Geometry: final body of the model. Coordinates: model frame, mm. A direction names the side the tool comes from. Coordinates: 2 decimals unless noted, no trailing zeros. Loops run counter-clockwise (first coordinate to the right, second up) from the corner with the lowest first, then second, coordinate; pieces in that order, holes last. Notation, with made-up numbers: (-24.5, 50) - (29.5, 50) arc R25 ccw to (29.5, 73) - close; hole circle Ø3 at (82, 30). An arc over 180 degrees is marked (long way). Put each result on its own line as item: value. Start each with the question number.
1) Reachability of faces 1 (the flat face through (-4, 4, -4)), 2 (the flat face through (0, 4, 17.5)) from +Z, -Z, +X, -X, +Y, -Y: full face, straight path, thin tool, end or side. Return the list, or none.
2) Material intervals for line 1 along Z through (x, y) = (13.5, 7); line 2 along Z through (x, y) = (-16, 5.75); line 3 along X through (y, z) = (3, -27), sorted ascending. Write a range as from..to.
3) Section C-C on x = -14.5. Output: boundary loops of the cut face in (y, z).
4) Draft query along X for faces 3 (the flat face through (-20, 4, -10)), 4 (the flat face through (20, 4, -10)), 5 (the cylindrical face through (-1.08, 1.97, -4.88)). Return one class per face: +X half, -X half, draft (parallel to the pull), parting line (faces both ways), or undercut.
5) Contact query for flat-ended pins moving along their axis: pin 1 Ø13.5 at (x, z) = (0.5, 1) entering from +Y; pin 2 Ø6 at (x, z) = (0, 0) entering from -Y. Output: stop coordinate, or through.
6) Section D-D on y = 6.75. Output: boundary loops of the cut face in (x, z).
7) Section B-B on x = 10. Output: boundary loops of the cut face in (y, z), and give its area (3 significant figures).
8) Section A-A on z = -14.5. Output: boundary loops of the cut face in (x, y).
```python
from build123d import *

# Parameters (mm, degrees)
F0_R     = 2.7
F0_R_2   = 1.7
F0_R_3   = 5
F1_DEPTH = 8
F2_R     = 8.5
F3_DEPTH = 4


with BuildPart() as f1:
    # F0 (on Front) → F1 (new body)
    with BuildSketch(Plane.XZ):
        with BuildLine():
            ThreePointArc((-18, 17.5), (-19.414214, 16.914214), (-20, 15.5))
            Line((-20, 15.5), (-20, -35.7))
            ThreePointArc((-20, -35.7), (-19.414214, -37.114214), (-18, -37.7))
            Line((-18, -37.7), (18, -37.7))
            ThreePointArc((18, -37.7), (19.414214, -37.114214), (20, -35.7))
            Line((20, -35.7), (20, 15.5))
            ThreePointArc((20, 15.5), (19.414214, 16.914214), (18, 17.5))
            Line((18, 17.5), (-18, 17.5))
        make_face()
        with Locations((-10, -27.7)):
            Circle(F0_R, mode=Mode.SUBTRACT)
        with Locations((-14.5, -14.5)):
            Circle(F0_R_2, mode=Mode.SUBTRACT)
        with Locations((10, -27.7)):
            Circle(F0_R, mode=Mode.SUBTRACT)
        with Locations((14.5, -14.5)):
            Circle(F0_R_2, mode=Mode.SUBTRACT)
        with Locations((-14.5, 14.5)):
            Circle(F0_R_2, mode=Mode.SUBTRACT)
        Circle(F0_R_3, mode=Mode.SUBTRACT)
        with Locations((14.5, 14.5)):
            Circle(F0_R_2, mode=Mode.SUBTRACT)
    extrude(amount=-F1_DEPTH)

    # F2 (on face) → F3 (cut)
    with BuildSketch(Plane(origin=(0, 8, 0), x_dir=(-1, 0, 0), z_dir=(0, 1, 0))):
        Circle(F2_R)
    extrude(amount=-F3_DEPTH, mode=Mode.SUBTRACT)


solid = f1.part
```
Answer block:
1. face 1: +Y
1. face 2: +Z, +X, -X, +Y, -Y
2. line 1: z = -37.7..-15.87, -13.13..13.13, 15.87..17.5
2. line 2: z = -37.7..-15.3, -13.7..13.7, 15.3..17.5
2. line 3: x = -20..-12.61, -7.39..7.39, 12.61..20
3. outline: (0, -37.7) - (8, -37.7) - (8, -16.2) - (0, -16.2) - close; (0, -12.8) - (8, -12.8) - (8, 12.8) - (0, 12.8) - close; (0, 16.2) - (8, 16.2) - (8, 17.5) - (0, 17.5) - close
4. face 3: -X half
4. face 4: +X half
4. face 5: undercut
5. pin 1: stops at y = 4
5. pin 2: passes through
6. outline: (-20, -35.7) arc R2 ccw to (-18, -37.7) - (18, -37.7) arc R2 ccw to (20, -35.7) - (20, 15.5) arc R2 ccw to (18, 17.5) - (-18, 17.5) arc R2 ccw to (-20, 15.5) - close; hole circle Ø3.4 at (-14.5, -14.5); hole circle Ø3.4 at (-14.5, 14.5); hole circle Ø5.4 at (-10, -27.7); hole circle Ø17 at (0, 0); hole circle Ø5.4 at (10, -27.7); hole circle Ø3.4 at (14.5, -14.5); hole circle Ø3.4 at (14.5, 14.5)
7. outline: (0, -37.7) - (8, -37.7) - (8, -30.4) - (0, -30.4) - close; (0, -25) - (8, -25) - (8, 17.5) - (0, 17.5) - close
7. area: 398 mm²
8. outline: (-20, 0) - (-16.2, 0) - (-16.2, 8) - (-20, 8) - close; (-12.8, 0) - (12.8, 0) - (12.8, 8) - (-12.8, 8) - close; (16.2, 0) - (20, 0) - (20, 8) - (16.2, 8) - close
